```python
from build123d import *

# Parameters (mm, degrees)
SKETCH_1_W          = 70
SKETCH_1_H          = 100
EXTRUDE_1_DEPTH     = 12
SKETCH_2_R          = 3
CUT_EXTRUDE_1_DEPTH = 10
SKETCH_3_R          = 3
CUT_EXTRUDE_2_DEPTH = 12
SKETCH_4_R          = 5.5
CUT_EXTRUDE_3_DEPTH = 6
CUT_EXTRUDE_START   = -10
SKETCH_5_R          = 3
CUT_EXTRUDE_4_DEPTH = 10
SKETCH_6_R          = 3
CUT_EXTRUDE_5_DEPTH = 10


with BuildPart() as part:
    # 草图1 → 凸台-拉伸1 (new body)
    with BuildSketch(Plane.XY):
        Rectangle(SKETCH_1_W, SKETCH_1_H)
    extrude(amount=EXTRUDE_1_DEPTH)

    # 草图2 → 切除-拉伸1 (cut)
    with BuildSketch(Plane.ZY.offset(35)):
        with Locations((6, -35)):
            Circle(SKETCH_2_R)
        with Locations((6, -15)):
            Circle(SKETCH_2_R)
        with Locations((6, 5)):
            Circle(SKETCH_2_R)
        with Locations((6, 25)):
            Circle(SKETCH_2_R)
    extrude(amount=-CUT_EXTRUDE_1_DEPTH, mode=Mode.SUBTRACT)

    # 草图3 → 切除-拉伸2 (cut)
    with BuildSketch(Plane.XY.offset(12)):
        with Locations((-29, 44)):
            Circle(SKETCH_3_R)
        with Locations((-9, 44)):
            Circle(SKETCH_3_R)
    extrude(amount=-CUT_EXTRUDE_2_DEPTH, mode=Mode.SUBTRACT)

    # 草图4 → 切除-拉伸3 (cut)
    with BuildSketch(Plane.XY.offset(12)):
        with Locations((-29, 44)):
            Circle(SKETCH_4_R)
        with Locations((-9, 44)):
            Circle(SKETCH_4_R)
    extrude(amount=-CUT_EXTRUDE_3_DEPTH, mode=Mode.SUBTRACT)

    # 草图5 → 切除-拉伸4 (cut)
    with BuildSketch(Plane(origin=(35, 0, 0), x_dir=(0, 0, -1), z_dir=(1, 0, 0)).offset(CUT_EXTRUDE_START)):
        with Locations(Location((-6, -35, 0), (0, 0, 180))):
            Circle(SKETCH_5_R)
        with Locations(Location((-6, -15, 0), (0, 0, 180))):
            Circle(SKETCH_5_R)
        with Locations(Location((-6, 5, 0), (0, 0, 180))):
            Circle(SKETCH_5_R)
        with Locations(Location((-6, 25, 0), (0, 0, 180))):
            Circle(SKETCH_5_R)
    extrude(amount=CUT_EXTRUDE_4_DEPTH, mode=Mode.SUBTRACT)

    # 草图6 → 切除-拉伸5 (cut)
    with BuildSketch(Plane.XZ.offset(50)):
        with Locations((-21, 6)):
            Circle(SKETCH_6_R)
        with Locations((-7, 6)):
            Circle(SKETCH_6_R)
        with Locations((7, 6)):
            Circle(SKETCH_6_R)
        with Locations((21, 6)):
            Circle(SKETCH_6_R)
    extrude(amount=-CUT_EXTRUDE_5_DEPTH, mode=Mode.SUBTRACT)


solid = part.part
```
Work out the finished part from the listing and answer in its coordinate system (mm). A direction names the side the tool comes from. Coordinates: 2 decimals unless noted, no trailing zeros. Loops run counter-clockwise (first coordinate to the right, second up) from the corner with the lowest first, then second, coordinate; pieces in that order, holes last. Notation, with made-up numbers: (-16, -29) - (-1, -29) arc R30 cw to (-1, -7) - close; hole circle Ø5 at (60, 61.25). An arc over 180 degrees is marked (long way). Use a Markdown table: item, result.
Item 1: Find section B-B, the plane x = 27.5. Determine the outline of the cut face in (y, z).
Evaluation:
| item | result |
|---|---|
| outline | (-50, 0) - (50, 0) - (50, 12) - (-50, 12) - close; hole circle Ø6 at (-35, 6); hole circle Ø6 at (-15, 6); hole circle Ø6 at (5, 6); hole circle Ø6 at (25, 6) |
Item 2: The mould has two halves that part along X. Classify faces 5 (the flat face through (25, -35, 6)), 6 (the cylindrical face through (-30.07, 23.85, 8.77)), 7 (the cylindrical face through (-31.21, 46.03, 3.04)): +X half, -X half, draft (parallel to the pull), parting line (faces both ways), or undercut.
Evaluation:
| item | result |
|---|---|
| face 5 | +X half |
| face 6 | draft |
| face 7 | undercut |
Item 3: Find section A-A, the plane x = -30. Determine the outline of the cut face in (y, z).
Evaluation:
| item | result |
|---|---|
| outline | (-50, 0) - (41.17, 0) - (41.17, 6) - (38.59, 6) - (38.59, 12) - (-50, 12) - close; (46.83, 0) - (50, 0) - (50, 12) - (49.41, 12) - (49.41, 6) - (46.83, 6) - close; hole circle Ø6 at (-35, 6); hole circle Ø6 at (-15, 6); hole circle Ø6 at (5, 6); hole circle Ø6 at (25, 6) |
Item 4: For faces 1 (the flat face through (-25, -15, 6)), 2 (the flat face through (-7, -40, 6)), 3 (the flat face through (25, 25, 6)), 4 (the flat face through (-26.6, 41.6, 6)), determine the directions among +Z, -Z, +X, -X, +Y, -Y from which every point of the face is accessible in a straight line to the end or side of a thin tool.
Evaluation:
| item | result |
|---|---|
| face 1 | -X |
| face 2 | -Y |
| face 3 | +X |
| face 4 | +Z |
Item 5: Find section D-D, the plane x = -11. Determine the outline of the cut face in (y, z), and give its area (3 significant figures).
Evaluation:
| item | result |
|---|---|
| outline | (-50, 0) - (41.76, 0) - (41.76, 6) - (38.88, 6) - (38.88, 12) - (-50, 12) - close; (46.24, 0) - (50, 0) - (50, 12) - (49.12, 12) - (49.12, 6) - (46.24, 6) - close |
| area | 1,110 mm2 |
Item 6: Find section C-C, the plane z = 10. Determine the outline of the cut face in (x, y).
Evaluation:
| item | result |
|---|---|
| outline | (-35, -50) - (35, -50) - (35, 50) - (-35, 50) - close; hole circle Ø11 at (-29, 44); hole circle Ø11 at (-9, 44) |
Item 7: Given pin 1 Ø3 at (y, z) = (25, 5.5) entering from +X; pin 2 Ø3 at (y, z) = (6, 7) entering from -X; pin 3 Ø3.5 at (x, z) = (21, 6) entering from -Y, each flat-ended and moving along its own axis, determine where each tip first touches the part or whether it passes through.
Evaluation:
| item | result |
|---|---|
| pin 1 | stops at x = 25 |
| pin 2 | stops at x = -25 |
| pin 3 | stops at y = -40 |
Item 8: Consider probe 1 along Y at (x, z) = (27.5, 6); probe 2 along Y at (x, z) = (-29, 8); probe 3 along Y at (x, z) = (-29, 4). Determine where each line is inside the solid, lowest interval first. Write a range as from..to.
Evaluation:
| item | result |
|---|---|
| probe 1 | y = -50..-38, -32..-18, -12..2, 8..22, 28..50 |
| probe 2 | y = -50..-37.24, -32.76..-17.24, -12.76..2.76, 7.24..22.76, 27.24..38.5, 49.5..50 |
| probe 3 | y = -50..-37.24, -32.76..-17.24, -12.76..2.76, 7.24..22.76, 27.24..41, 47..50 |
